Read the model definition and answer for the solid it produces. Units are mm, in the model's axes. Face numbers are marked on the shaded views. A direction names the side the tool comes from. Round coordinates to 2 decimals unless told otherwise and drop trailing zeros. Order: outer loops, then holes, each group sorted by start corner. A loop starts at its lowest first (then second) coordinate and runs counter-clockwise, first axis right, second up. Notation, with made-up numbers: (85, 47.5) - (116, 47.5) arc R21 ccw to (116, 72.5) - close; hole circle Ø1 at (21, -9.75). An arc over 180 degrees is marked (long way). One line per question, with ' | ' between items. Start each with the question number.
1) The part is cut by section A-A, the plane y = -31. Give the vertices of the cut face in (x, z).
2) For the marked faces 1 and 2, determine the directions among +Z, -Z, +X, -X, +Y, -Y from which every point of the face is accessible in a straight line to the end or side of a thin tool.
3) The part is cut by section B-B, the plane y = -37.5. Give the vertices of the cut face in (x, z), plus the area to 3 significant figures.
4) Straight lines are drawn through the part: line 1 (Z direction, x = 2.25, y = -14.5); line 2 (Y direction, x = 1, z = -158); line 3 (Y direction, x = 1.25, z = -57). For each, find the intervals that lie inside material, in ascending order. Write a range as from..to.
5) Flat-ended cylindrical pins translate along their axes: pin 1 (3 mm diameter, centred on x = 4.5, y = -50, fed in from +Z); pin 2 (1.9 mm diameter, centred on x = 3, y = -17.5, fed in from -Z). Find the tip coordinate at first contact, or state that the pin passes through.
6) The mould has two halves that part along Y. Classify the marked faces 3 and 4: pulls with the +Y half, pulls with the -Y half, needs draft (parallel to the pull), parting line crosses it, or undercut.
from build123d import *

# Parameters (mm, degrees)
BOSS_EXTRUDE1_DEPTH = 6.35
CUT_EXTRUDE1_DEPTH  = 178.004470283
CUT_EXTRUDE2_DEPTH  = 1.27


with BuildPart() as part:
    # Sketch1 → Boss-Extrude1 (new body)
    with BuildSketch(Plane(origin=(0, 0, 0), x_dir=(0, 0, -1), z_dir=(1, 0, 0))):
        Polygon((0, 0), (165.1, 0), (165.1, -14.859), (158.75, -14.859), (158.75, -12.319), (154.94, -12.319), (154.94, -14.859), (152.4, -14.859), (152.4, -18.669), (154.94, -18.669), (154.94, -21.209), (158.75, -21.209), (158.75, -18.669), (165.1, -18.669), (165.1, -44.831), (158.75, -44.831), (158.75, -42.291), (154.94, -42.291), (154.94, -44.831), (152.4, -44.831), (152.4, -48.641), (154.94, -48.641), (154.94, -51.181), (158.75, -51.181), (158.75, -48.641), (165.1, -48.641), (165.1, -63.5), (0, -63.5), (0, -48.641), (6.35, -48.641), (6.35, -51.181), (10.16, -51.181), (10.16, -48.641), (12.7, -48.641), (12.7, -44.831), (10.16, -44.831), (10.16, -42.291), (6.35, -42.291), (6.35, -44.831), (0, -44.831), (0, -18.669), (6.35, -18.669), (6.35, -21.209), (10.16, -21.209), (10.16, -18.669), (12.7, -18.669), (12.7, -14.859), (10.16, -14.859), (10.16, -12.319), (6.35, -12.319), (6.35, -14.859), (0, -14.859), align=None)
    extrude(amount=BOSS_EXTRUDE1_DEPTH)

    # Sketch2 → Cut-Extrude1 (cut, through all)
    with BuildSketch(Plane(origin=(6.35, 0, 0), x_dir=(0, 0, -1), z_dir=(1, 0, 0))):
        Polygon((50.927, -63.5), (54.737, -63.5), (54.737, -57.15), (57.277, -57.15), (57.277, -53.34), (54.737, -53.34), (54.737, -50.8), (50.927, -50.8), (50.927, -53.34), (48.387, -53.34), (48.387, -57.15), (50.927, -57.15), align=None)
        Polygon((110.363, -63.5), (114.173, -63.5), (114.173, -57.15), (116.713, -57.15), (116.713, -53.34), (114.173, -53.34), (114.173, -50.8), (110.363, -50.8), (110.363, -53.34), (107.823, -53.34), (107.823, -57.15), (110.363, -57.15), align=None)
    extrude(amount=-CUT_EXTRUDE1_DEPTH, mode=Mode.SUBTRACT)

    # Sketch3 → Cut-Extrude2 (cut)
    with BuildSketch(Plane(origin=(6.35, 0, 0), x_dir=(0, 0, -1), z_dir=(1, 0, 0))):
        Polygon((82.55, -20.32), (78.792923653, -28.377076227), (69.902923653, -28.377076227), (76.713058752, -34.091458077), (74.412157441, -42.678538673), (82.55, -39.09976535), (90.687842559, -42.678538673), (88.386941248, -34.091458077), (95.197076347, -28.377076227), (86.307076347, -28.377076227), align=None)
        Polygon((25.4635, -20.32), (21.706423653, -28.377076227), (12.816423653, -28.377076227), (19.626558752, -34.091458077), (17.325657441, -42.678538673), (25.4635, -39.09976535), (33.601342559, -42.678538673), (31.300441248, -34.091458077), (38.110576347, -28.377076227), (29.220576347, -28.377076227), align=None)
        Polygon((139.6365, -20.32), (135.879423653, -28.377076227), (126.989423653, -28.377076227), (133.799558752, -34.091458077), (131.498657441, -42.678538673), (139.6365, -39.09976535), (147.774342559, -42.678538673), (145.473441248, -34.091458077), (152.283576347, -28.377076227), (143.393576347, -28.377076227), align=None)
    extrude(amount=-CUT_EXTRUDE2_DEPTH, mode=Mode.SUBTRACT)


solid = part.part
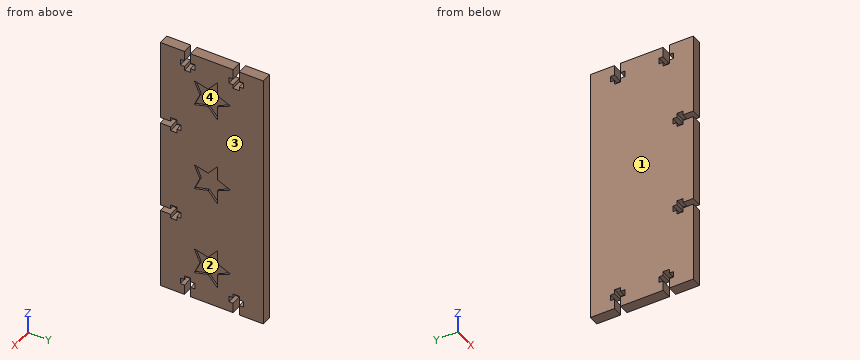
Values:
1) outline: (0, -165.1) - (6.35, -165.1) - (6.35, -149.16) - (5.08, -149.16) - (5.08, -130.12) - (6.35, -130.12) - (6.35, -92.07) - (5.08, -92.07) - (5.08, -73.03) - (6.35, -73.03) - (6.35, -34.98) - (5.08, -34.98) - (5.08, -15.94) - (6.35, -15.94) - (6.35, 0) - (0, 0) - close
2) face 1: +Z, -Z, -X, +Y, -Y | face 2: +X
3) outline: (0, -165.1) - (6.35, -165.1) - (6.35, -146.39) - (5.08, -146.39) - (5.08, -132.89) - (6.35, -132.89) - (6.35, -89.3) - (5.08, -89.3) - (5.08, -75.8) - (6.35, -75.8) - (6.35, -32.21) - (5.08, -32.21) - (5.08, -18.71) - (6.35, -18.71) - (6.35, 0) - (0, 0) - close | area: 997 mm^2
4) line 1: z = -165.1..-158.75, -154.94..-10.16, -6.35..0 | line 2: y = -63.5..-51.18, -42.29..-21.21, -12.32..0 | line 3: y = -63.5..-57.15, -53.34..0
5) pin 1: stops at z = 0 | pin 2: stops at z = -152.4
6) face 3: needs draft | face 4: undercut
